Source: CAD feature listing. Evaluate the final solid. Frame: model axes, mm. Face numbers are marked on the shaded views. Coordinates: 2 decimals unless noted, no trailing zeros. Loops run counter-clockwise (first coordinate to the right, second up) from the corner with the lowest first, then second, coordinate; pieces in that order, holes last.
Item 1: Section query D-D, the plane x = -3. Return the cut outline in (y, z), then the cut area to 3 significant figures.
Item 2: Section query C-C, the plane z = 0.75. State how many separate pieces and enclosed holes the cut face has, then the cut area to 3 significant figures.
Item 3: Section query B-B, the plane y = -8.5. Return the cut outline in (x, z).
Item 4: Section query A-A, the plane x = 0. Return the cut outline in (y, z), then the cut area to 3 significant figures.
Item 5: Line query: probe 1 along Y at (x, z) = (0, 0.2); probe 2 along Y at (x, z) = (4, 0.65); probe 3 along Y at (x, z) = (2, 0.45). Output: solid intervals per line, ascending.
Item 6: Pull-direction query (Y, two-part tool) for the marked faces 1, 2 and 3; classes: +Y half, -Y half, draft (parallel to the pull), parting line (faces both ways), or undercut.
```python
from build123d import *

# Parameters (mm, degrees)
SKETCH1_R           = 0.5
BOSS_EXTRUDE2_DEPTH = 1
FILLET2_R           = 0.2
SKETCH3_R           = 0.25
CUT_EXTRUDE1_DEPTH  = 1
SKETCH4_R           = 0.25
CUT_EXTRUDE2_DEPTH  = 1


with BuildPart() as part:
    # Sketch1 → Boss-Extrude2 (new body)
    with BuildSketch(Plane.XY):
        with BuildLine():
            Line((4.5, -9), (0, -9))
            Line((0, -9), (-4.5, -9))
            Line((-4.5, -9), (-4.5, -0.866025404))
            ThreePointArc((-4.5, -0.866025404), (-5, 0), (-4.5, 0.866025404))
            ThreePointArc((-4.5, 0.866025404), (-5.008977866, 3.264145238), (-4.356520714, 5.627265394))
            ThreePointArc((-4.356520714, 5.627265394), (-4.888888889, 7.01967566), (-3.445948422, 7.394035154))
            ThreePointArc((-3.445948422, 7.394035154), (0, 9), (3.445948422, 7.394035154))
            ThreePointArc((3.445948422, 7.394035154), (4.888888889, 7.01967566), (4.356520714, 5.627265394))
            ThreePointArc((4.356520714, 5.627265394), (4.997611441, 3.263802712), (4.5, 0.866025404))
            ThreePointArc((4.5, 0.866025404), (5, 0), (4.5, -0.866025404))
            Line((4.5, -0.866025404), (4.5, -9))
        make_face()
        with Locations((-4, 0)):
            Circle(SKETCH1_R, mode=Mode.SUBTRACT)
        with Locations((-4, 6.561552813)):
            Circle(SKETCH1_R, mode=Mode.SUBTRACT)
        with Locations(Location((4, 6.561552813, 0), (0, 0, 180))):
            Circle(SKETCH1_R, mode=Mode.SUBTRACT)
        with Locations(Location((4, 0, 0), (0, 0, 180))):
            Circle(SKETCH1_R, mode=Mode.SUBTRACT)
    extrude(amount=BOSS_EXTRUDE2_DEPTH)

    # Fillet2
    fillet2_edges = [part.edges().sort_by_distance(p)[0] for p in [
        (-4.5, -9, 0.5),
        (-4.5, -0.866025404, 0.5),
        (-4.5, 0.866025404, 0.5),
        (-4.356520714, 5.627265394, 0.5),
        (-3.445948422, 7.394035154, 0.5),
        (3.445948422, 7.394035154, 0.5),
        (4.356520714, 5.627265394, 0.5),
        (4.5, 0.866025404, 0.5),
        (4.5, -0.866025404, 0.5),
        (4.5, -9, 0.5),
    ]]
    fillet(fillet2_edges, radius=FILLET2_R)

    # Sketch3 → Cut-Extrude1 (cut)
    with BuildSketch(Plane(origin=(0, 0, 0), x_dir=(-1, 0, 0), z_dir=(0, 0, -1))):
        with Locations((3.839007705, 3.108348927)):
            Circle(SKETCH3_R)
        with Locations((1.839007705, -0.355752688)):
            Circle(SKETCH3_R)
        with Locations((-2.160992295, -0.355752688)):
            Circle(SKETCH3_R)
        with Locations((-4.160992295, 3.108348927)):
            Circle(SKETCH3_R)
        with Locations((-2.160992295, 6.572450542)):
            Circle(SKETCH3_R)
        with Locations((1.839007705, 6.572450542)):
            Circle(SKETCH3_R)
    extrude(amount=-CUT_EXTRUDE1_DEPTH, mode=Mode.SUBTRACT)

    # Sketch4 → Cut-Extrude2 (cut)
    with BuildSketch(Plane(origin=(0, 0, 0), x_dir=(-1, 0, 0), z_dir=(0, 0, -1))):
        with Locations((4, -1.5)):
            Circle(SKETCH4_R)
        with Locations((4, -8.5)):
            Circle(SKETCH4_R)
        with Locations((0, -1.5)):
            Circle(SKETCH4_R)
        with Locations((0, -8.5)):
            Circle(SKETCH4_R)
    extrude(amount=-CUT_EXTRUDE2_DEPTH, mode=Mode.SUBTRACT)


solid = part.part
```
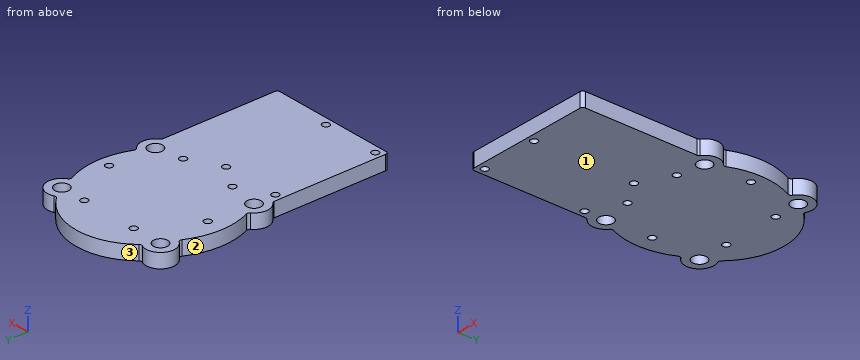
Verdict:
1. outline: (-9, 0) - (7.85, 0) - (7.85, 1) - (-9, 1) - close
1. area: 16.9 mm2
2. separate pieces: 1
2. enclosed holes: 14
2. area: 156 mm2
3. outline: (-4.5, 0) - (-4.25, 0) - (-4.25, 1) - (-4.5, 1) - close; (-3.75, 0) - (-0.25, 0) - (-0.25, 1) - (-3.75, 1) - close; (0.25, 0) - (4.5, 0) - (4.5, 1) - (0.25, 1) - close
4. outline: (-9, 0) - (-8.75, 0) - (-8.75, 1) - (-9, 1) - close; (-8.25, 0) - (-1.75, 0) - (-1.75, 1) - (-8.25, 1) - close; (-1.25, 0) - (9, 0) - (9, 1) - (-1.25, 1) - close
4. area: 17.0 mm2
5. probe 1: y = -9 to -8.75, -8.25 to -1.75, -1.25 to 9
5. probe 2: y = -9 to -0.5, 0.5 to 2.92, 3.3 to 6.06, 7.06 to 7.56
5. probe 3: y = -9 to -0.55, -0.16 to 6.38, 6.76 to 8.53
6. face 1: draft
6. face 2: undercut
6. face 3: +Y half
